Autodesk Inventor part; units mm, degrees
ref_plane "YZ Plane" through (0, 0, 0) normal (1, 0, 0) x (0, 1, 0)
ref_plane "XZ Plane" through (0, 0, 0) normal (0, 1, 0) x (-1, 0, 0)
ref_plane "XY Plane" through (0, 0, 0) normal (0, 0, 1) x (1, 0, 0)
sketch "Skizze1" plane through (0, 0, 0) normal (1, 0, 0) x (0, 1, 0)
  line L0 (0, 0) -> (3, 0)
  line L1 (3, 0) -> (3, -19)
  arc A0 (-3, -19) -> (3, -19) centre (0, -19) ccw
  line L2 (-3, -19) -> (0, 0)
  dimension "d0" = 3
  dimension "d1" = 19
  dimension "d2" = 3
  dimension "d3" = 3
extrude "Extrusion1" add sketch "Skizze1" along normal blind 3
sketch "Skizze2" plane through (3, 0, 0) normal (1, 0, 0) x (0, 0, -1)
  arc A0 (19, -3) -> (19, 3) centre (19, 0) ccw
  point P0 (0, 0)
hole "Bohrung1" at (3, 0, -19) direction (-1, 0, 0) diameter 3 depth 3
properties part number "109 part 2"
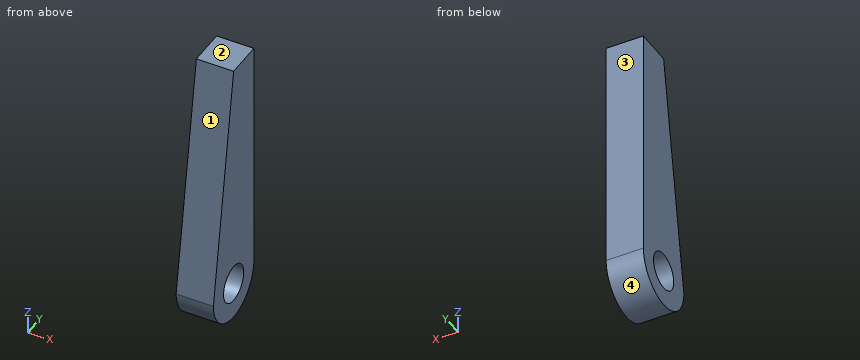
Could you check a few things on this model? Use its own coordinates, in mm. Face numbers are marked on the shaded views. Coordinates: 2 decimals unless noted, no trailing zeros. Order: outer loops, then holes, each group sorted by start corner. A loop starts at its lowest first (then second) coordinate and runs counter-clockwise, first axis right, second up. Notation, with made-up numbers: M 44,11.25 L 66,11.25 A14 ccw 66,38.25 Z; hole C 32.5,54 d6. An arc over 180 degrees is marked long. Use one line per item in the form item = value. Start each with the question number.
1. For pin 1 (1.5 mm diameter, centred on x = 2.5, z = -12, fed in from -Y), with a flat end and sliding along its axis, tell me the tip position at first contact or that it passes through.
2. We'd pull the mould along Y, two halves only. Please class the marked faces 1, 2, 3 and 4: +Y half, -Y half, draft (parallel to the pull), parting line (faces both ways), or undercut.
3. Please list where these lines run through material, in increasing order: line 1 (Y direction, x = 2.35, z = -19); line 2 (Y direction, x = 1.45, z = -19.75); line 3 (Z direction, x = 2.55, y = 0.6).
4. Suppose I cut it at C-C on z = -6.75. Write out the boundary of the cut face in (x, y).
5. Suppose I cut it at B-B on z = -9.5. Write out the boundary of the cut face in (x, y), then the cut area to 3 significant figures.
6. Suppose I cut it at A-A on x = 1.2. Write out the boundary of the cut face in (y, z).
Geometry says:
q1.pin_1 = -2.01
q2.face_1 = -Y half
q2.face_2 = draft
q2.face_3 = +Y half
q2.face_4 = parting line
q3.line_1 = -3 to -1.5, 1.5 to 3
q3.line_2 = -2.9 to -1.3, 1.3 to 2.9
q3.line_3 = -21.94 to -20.37, -17.63 to 0
q4.outline = M 0,-1.07 L 3,-1.07 L 3,3 L 0,3 Z
q5.outline = M 0,-1.5 L 3,-1.5 L 3,3 L 0,3 Z
q5.area = 13.5 mm^2
q6.outline = M -3,-19 A3 ccw 3,-19 L 3,0 L 0,0 Z; hole C 0,-19 d3
